Input: part model. Units: mm. Frame: model coordinates. A direction names the side the tool comes from. Round coordinates to 2 decimals unless told otherwise and drop trailing zeros. Order: outer loops, then holes, each group sorted by start corner. A loop starts at its lowest first (then second) coordinate and runs counter-clockwise, first axis right, second up.
Item 1: First-contact query: pin 1 (3 mm diameter, centred on x = 13.5, z = -2.5, fed in from -Y); pin 2 (6 mm diameter, centred on y = 8.5, z = -10, fed in from +X); pin 3 (6.5 mm diameter, centred on y = 6.5, z = -13.5, fed in from +X); pin 4 (1 mm diameter, centred on x = 14.5, y = 12.5, fed in from -Z). Flat tips, straight axial feed; report the tip coordinate or a pass-through.
Item 2: Cut plane A-A on y = 8.5. Output: boundary loops of the cut face in (x, z), then the cut area to 3 significant figures.
Item 3: Cut plane D-D on x = 5. Output: boundary loops of the cut face in (y, z), then the cut area to 3 significant figures.
Item 4: Reachability of faces 1 (the flat face through (13, 11, -2)), 2 (the flat face through (20, 8, -1)) from +Z, -Z, +X, -X, +Y, -Y: full face, straight path, thin tool, end or side. Return the list, or none.
Item 5: Cut plane C-C on z = -10. Output: boundary loops of the cut face in (x, y), then the cut area to 3 significant figures.
Item 6: Mould query, pull axis Y, two halves, no side actions, for faces 3 (the cylindrical face through (0.986, 8.643, -6.753)), 4 (the flat face through (8, 17, -8)), 5 (the flat face through (8, 0, -8)), 6 (the flat face through (10, 12, 0)). Classes: released by +Y, released by -Y, zero draft, split by the parting line, or undercut.
Item 7: Cut plane B-B on x = 10. Output: boundary loops of the cut face in (y, z), then the cut area to 3 significant figures.
Item 8: Line query: L1, parallel to Y at x = 10, z = -0.7; L2, parallel to Y at x = 10, z = -10; L3, parallel to Z at x = 18.5, y = 9.75. Output: solid intervals per line, ascending.
```python
from build123d import *

# Parameters (mm, degrees)
SKETCH1_W           = 20
SKETCH1_H           = 17
SKETCH1_R           = 3.25
BOSS_EXTRUDE1_DEPTH = 2
SKETCH2_W           = 20
SKETCH2_H           = 17
SKETCH2_R           = 3.25
BOSS_EXTRUDE2_DEPTH = 2
BOSS_EXTRUDE3_DEPTH = 2
BOSS_EXTRUDE4_DEPTH = 2


with BuildPart() as part:
    # Sketch1 → Boss-Extrude1 (new body)
    with BuildSketch(Plane.XY):
        with Locations((10, 8.5)):
            Rectangle(SKETCH1_W, SKETCH1_H)
        with Locations((10, 8.5)):
            Circle(SKETCH1_R, mode=Mode.SUBTRACT)
    extrude(amount=-BOSS_EXTRUDE1_DEPTH)

    # Sketch2 → Boss-Extrude2 (add)
    with BuildSketch(Plane(origin=(0, 0, 0), x_dir=(0, 0, -1), z_dir=(1, 0, 0))):
        with Locations((10, 8.5)):
            Rectangle(SKETCH2_W, SKETCH2_H)
        with Locations((10, 8.5)):
            Circle(SKETCH2_R, mode=Mode.SUBTRACT)
    extrude(amount=BOSS_EXTRUDE2_DEPTH)

    # Sketch3 → Boss-Extrude3 (add)
    with BuildSketch(Plane(origin=(0, 17, 0), x_dir=(1, 0, 0), z_dir=(0, 1, 0))):
        Polygon((2, 20), (20, 2), (2, 2), align=None)
    extrude(amount=-BOSS_EXTRUDE3_DEPTH)

    # Sketch4 → Boss-Extrude4 (add)
    with BuildSketch(Plane.XZ):
        Polygon((2, -20), (20, -2), (2, -2), align=None)
    extrude(amount=-BOSS_EXTRUDE4_DEPTH)


solid = part.part
```
From the geometry:
1. pin 1: stops at y = 0
1. pin 2: passes through
1. pin 3: stops at x = 2
1. pin 4: stops at z = -2
2. outline: (0, -20) - (2, -20) - (2, -13.25) - (0, -13.25) - close; (0, -6.75) - (2, -6.75) - (2, -2) - (6.75, -2) - (6.75, 0) - (0, 0) - close; (13.25, -2) - (20, -2) - (20, 0) - (13.25, 0) - close
2. area: 50.0 mm2
3. outline: (0, -17) - (2, -17) - (2, -2) - (15, -2) - (15, -17) - (17, -17) - (17, 0) - (0, 0) - close
3. area: 94.0 mm2
4. face 1: -Z, +X
4. face 2: +Z, -Z, +X, +Y, -Y
5. outline: (0, 0) - (12, 0) - (12, 2) - (2, 2) - (2, 5.25) - (0, 5.25) - close; (0, 11.75) - (2, 11.75) - (2, 15) - (12, 15) - (12, 17) - (0, 17) - close
5. area: 61.0 mm2
6. face 3: undercut
6. face 4: released by +Y
6. face 5: released by -Y
6. face 6: zero draft
7. outline: (0, -12) - (2, -12) - (2, -2) - (5.25, -2) - (5.25, 0) - (0, 0) - close; (11.75, -2) - (15, -2) - (15, -12) - (17, -12) - (17, 0) - (11.75, 0) - close
7. area: 61.0 mm2
8. L1: y = 0 to 5.25, 11.75 to 17
8. L2: y = 0 to 2, 15 to 17
8. L3: z = -2 to 0
